Could you check a few things on this model? Use its own coordinates, in mm. Give positions to 0.01 mm unless a question says otherwise; leave off trailing zeros. Loops run counter-clockwise (first coordinate to the right, second up) from the corner with the lowest first, then second, coordinate; pieces in that order, holes last. Notation, with made-up numbers: M 61.5,36.5 L 103.5,36.5 A19 cw 103.5,59.5 Z; hole C -29.5,1.25 d8. An arc over 180 degrees is marked long. Write each question's results on one line, items separated by ' | '. Start each with the question number.
from build123d import *

# Parameters (mm, degrees)
F1_DEPTH = 1219.2
F2_R     = 4.7625
F3_DEPTH = 31.751
F4_R     = 4.7625
F5_DEPTH = 25.4


with BuildPart() as f1:
    # F0 (on Top) → F1 (new body)
    with BuildSketch(Plane.XY):
        Polygon((0, 6.35), (0, 0), (31.75, 0), (31.75, 31.75), (25.4, 31.75), (25.4, 6.35), align=None)
    extrude(amount=F1_DEPTH)

    # F2 (on face) → F3 (cut, through all)
    with BuildSketch(Plane.YZ.offset(31.75)):
        with Locations((15.875, 12.7)):
            Circle(F2_R)
    extrude(amount=-F3_DEPTH, mode=Mode.SUBTRACT)

    # F4 (on face) → F5 (join)
    with BuildSketch(Plane.YZ.offset(31.75)):
        with Locations((15.875, 508)):
            Circle(F4_R)
    extrude(amount=F5_DEPTH)


solid = f1.part
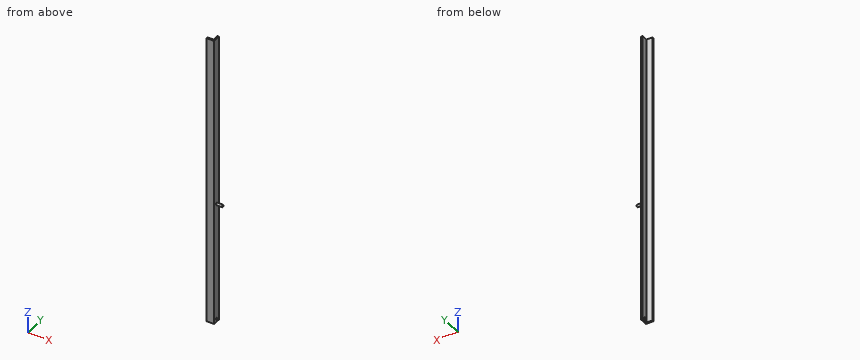
1) I'm going to push flat-ended pins straight in: P1, Ø9.5, axis at y = 12, z = 534, coming from the +X side; P2, Ø12, axis at y = 19.5, z = 928, coming from the -X side; P3, Ø12, axis at x = 15, z = 645.5, coming from the +Y side. Where does each tip first touch, or does it pass through?
2) If we section it at A-A on z = 106.5: Write out the boundary of the cut face in (x, y), plus the area to 3 significant figures.
3) Please list where these lines run through material, in increasing order: line 1 (Z direction, x = 30, y = 15.5); line 2 (X direction, y = 16.5, z = 861); line 3 (Y direction, x = 24.5, z = 852.5). Write a range as from..to.
4) If we section it at B-B on x = 46: Write out the boundary of the cut face in (y, z) (1 decimal).
Calculated:
1) P1: stops at x = 31.75 | P2: stops at x = 25.4 | P3: stops at y = 6.35
2) outline: M 0,0 L 31.75,0 L 31.75,31.75 L 25.4,31.75 L 25.4,6.35 L 0,6.35 Z | area: 363 mm2
3) line 1: z = 0..7.95, 17.45..1219.2 | line 2: x = 25.4..31.75 | line 3: y = 0..6.35
4) outline: C 15.9,508 d9.5
